```python
from build123d import *

# Parameters (mm, degrees)
F0_W     = 75
F0_H     = 75
F0_W_2   = 71
F0_H_2   = 71
F1_DEPTH = 70
F2_R     = 5
F3_T     = -2
F6_DEPTH = 5


with BuildPart() as f1:
    # F0 (on Top) → F1 (new body)
    with BuildSketch(Plane.XY):
        Rectangle(F0_W, F0_H)
        Rectangle(F0_W_2, F0_H_2, mode=Mode.SUBTRACT)
        Rectangle(F0_W_2, F0_H_2)
    extrude(amount=F1_DEPTH)

    # F2
    f2_edges = [f1.edges().sort_by_distance(p)[0] for p in [
        (-37.5, -37.5, 35),
        (37.5, -37.5, 35),
        (0, -37.5, 0),
        (-37.5, 0, 0),
        (-37.5, 37.5, 35),
        (0, 37.5, 0),
        (37.5, 37.5, 35),
        (37.5, 0, 0),
    ]]
    fillet(f2_edges, radius=F2_R)

    # F3
    f3_openings = [f1.faces().sort_by_distance(p)[0] for p in [
        (0, 0, 70),
    ]]
    offset(amount=F3_T, openings=f3_openings)

    # F5 (on offset) → F6 (cut)
    with BuildSketch(Plane.XY.offset(70)):
        with BuildLine():
            Line((-36.5, 32.5), (-36.5, -32.5))
            ThreePointArc((-36.5, -32.5), (-35.3284271247, -35.3284271247), (-32.5, -36.5))
            Line((-32.5, -36.5), (32.5, -36.5))
            ThreePointArc((32.5, -36.5), (35.3284271247, -35.3284271247), (36.5, -32.5))
            Line((36.5, -32.5), (36.5, 32.5))
            ThreePointArc((36.5, 32.5), (35.3284271247, 35.3284271247), (32.5, 36.5))
            Line((32.5, 36.5), (-32.5, 36.5))
            ThreePointArc((-32.5, 36.5), (-35.3284271247, 35.3284271247), (-36.5, 32.5))
        make_face()
    extrude(amount=-F6_DEPTH, mode=Mode.SUBTRACT)


solid = f1.part
```
Work out the finished part from the listing and answer in its coordinate system (mm). A direction names the side the tool comes from. Round coordinates to 2 decimals unless told otherwise and drop trailing zeros. Write each loop counter-clockwise with the first axis right and the second up, starting at its lowest first coordinate (ties: lowest second). Pieces come first, ordered by that corner, then holes. Notation, with made-up numbers: (1.5, -39.5) - (30.5, -39.5) arc R13 ccw to (30.5, -34.5) - close; hole circle Ø11 at (-2.75, -13.5). An arc over 180 degrees is marked (long way). Return JSON: item names as keys, results as strings. Group by question number.
Q1. The part is cut by section A-A on y = 25. Write down the section's boundary in (x, z), then the cut area to 3 significant figures.
Q2. This flat-tipped pin is pushed along its axis until it touches: pin 1 Ø4 at (x, y) = (-17, -16) entering from +Z. Where does it stop, or does it pass through?
Q3. For faces 1 (the flat face through (0, -37.5, 37)), 2 (the flat face through (-35.5, 0, 35)), determine the directions among +Z, -Z, +X, -X, +Y, -Y from which every point of the face is accessible in a straight line to the end or side of a thin tool.
Q4. The part is cut by section B-B on z = 39.5. Write down the section's boundary in (x, y), then the cut area to 3 significant figures.
Q5. Find the intervals of material crossed by L1, parallel to X at y = 3, z = 28; L2, parallel to Y at x = -31.5, z = 67, in increasing order.
Q6. The mould has two halves that part along X. Classify faces 3 (the cylindrical face through (0.45, -36.07, 1.5)), 4 (the cylindrical face through (0.45, 34.64, 2.9)), 5 (the cylindrical face through (36.07, 36, 37.96)): released by +X, released by -X, zero draft, split by the parting line, or undercut.
Solved:
{
 "1": {"outline": "(-37.5, 5) arc R5 ccw to (-32.5, 0) - (32.5, 0) arc R5 ccw to (37.5, 5) - (37.5, 70) - (36.5, 70) - (36.5, 65) - (35.5, 65) - (35.5, 5) arc R3 cw to (32.5, 2) - (-32.5, 2) arc R3 cw to (-35.5, 5) - (-35.5, 65) - (-36.5, 65) - (-36.5, 70) - (-37.5, 70) - close", "area": "405 mm²"},
 "2": {"pin 1": "z = 2"},
 "3": {"face 1": "+Z, -Z, +X, -X, -Y", "face 2": "+Z"},
 "4": {"outline": "(-37.5, -32.5) arc R5 ccw to (-32.5, -37.5) - (32.5, -37.5) arc R5 ccw to (37.5, -32.5) - (37.5, 32.5) arc R5 ccw to (32.5, 37.5) - (-32.5, 37.5) arc R5 ccw to (-37.5, 32.5) - close; hole (-35.5, -32.5) arc R3 ccw to (-32.5, -35.5) - (32.5, -35.5) arc R3 ccw to (35.5, -32.5) - (35.5, 32.5) arc R3 ccw to (32.5, 35.5) - (-32.5, 35.5) arc R3 ccw to (-35.5, 32.5) - close", "area": "570 mm²"},
 "5": {"L1": "-37.5 to -35.5, 35.5 to 37.5", "L2": "-37.5 to -36.5, 36.5 to 37.5"},
 "6": {"face 3": "zero draft", "face 4": "undercut", "face 5": "released by +X"}
}
